from build123d import *

# Parameters (mm, degrees)
SKETCH1_R           = 2.39
SKETCH1_R_2         = 2.032
BOSS_EXTRUDE1_DEPTH = 3.175
FILLET1_R           = 9.525


with BuildPart() as part:
    # Sketch1 → Boss-Extrude1 (new body)
    with BuildSketch(Plane.XY):
        Polygon((-13.549562782, 51.201238591), (55.395997605, -32.358681046), (47.399630983, -77.865858829), (-38.635835903, 26.208991527), align=None)
        with Locations((-26.780789006, 24.707545021)):
            Circle(SKETCH1_R, mode=Mode.SUBTRACT)
        with Locations((24.186660888, -13.868436177)):
            Circle(SKETCH1_R_2, mode=Mode.SUBTRACT)
        with Locations((19.493324021, -31.017809025)):
            Circle(SKETCH1_R_2, mode=Mode.SUBTRACT)
        with Locations((39.76308397, -33.93171218)):
            Circle(SKETCH1_R_2, mode=Mode.SUBTRACT)
        with Locations((35.069747103, -51.081085027)):
            Circle(SKETCH1_R_2, mode=Mode.SUBTRACT)
    extrude(amount=BOSS_EXTRUDE1_DEPTH)

    # Fillet1
    fillet1_edges = [part.edges().sort_by_distance(p)[0] for p in [
        (-13.549562782, 51.201238591, 1.5875),
        (55.395997605, -32.358681046, 1.5875),
        (47.399630983, -77.865858829, 1.5875),
        (-38.635835903, 26.208991527, 1.5875),
    ]]
    fillet(fillet1_edges, radius=FILLET1_R)


solid = part.part
Verification items for the finished model (mm, model axes). Give positions to 0.01 mm unless a question says otherwise; leave off trailing zeros. Order: outer loops, then holes, each group sorted by start corner. A loop starts at its lowest first (then second) coordinate and runs counter-clockwise, first axis right, second up. Notation, with made-up numbers: M 74,32.25 L 79,32.25 A22 ccw 79,57.25 Z; hole C -1.75,-18 d1. An arc over 180 degrees is marked long. Answer as a JSON object with one key per item and string values. Group by question number.
1) Depth check by flat-ended pin: pin 1 Ø3.5 at (x, y) = (19.49, -31.02) entering from +Z; pin 2 Ø1.5 at (y, z) = (32, 2.5) entering from +X; pin 3 Ø1 at (x, z) = (7.5, 2.5) entering from +Y; pin 4 Ø6.5 at (x, y) = (39.76, -33.93) entering from +Z (3 decimals). Enter the tip coordinate at first touch or a pass-through.
2) Cross-section at B-B (y = -2). Enter the section's corners in (x, z) (3 decimals).
3) Cross-section at A-A (z = 2.4). Enter the section's corners in (x, y) (3 decimals), then the cut area to 3 significant figures.
4) Mould release check, pull along X, two halves, no side actions. Record for faces 1 (the face through (-13.664, 46.577, 1.61)), 2 (the face through (1.043, -21.79, 1.565)), 3 (the face through (20.43, -32.82, 1.57)): released by +X, released by -X, zero draft, split by the parting line, or undercut.
5) Scan lines: line 1 along X through (y, z) = (-13.5, 2.5); line 2 along X through (y, z) = (-14.5, 1.2); line 3 along X through (y, z) = (-24.5, 1.8). Record each from-to range of solid material in increasing order. Write a range as [from, to].
6) Cross-section at C-C (x = 14). Enter the section's corners in (y, z) (3 decimals).
Result sheet:
{
 "1": {"pin 1": "passes through", "pin 2": "stops at x = 2.91", "pin 3": "stops at y = 26.3", "pin 4": "stops at z = 3.175"},
 "2": {"outline": "M -15.316,0 L 30.347,0 L 30.347,3.175 L -15.316,3.175 Z"},
 "3": {"outline": "M -33.105,19.519 L 34.249,-61.958 A9.525 ccw 50.972,-57.538 L 54.636,-36.683 A9.525 ccw 52.602,-28.972 L -6.891,43.132 A9.525 ccw -20.961,43.818 L -32.486,32.335 A9.525 ccw Z; hole C -26.781,24.708 d4.78; hole C 19.493,-31.018 d4.064; hole C 24.187,-13.868 d4.064; hole C 35.07,-51.081 d4.064; hole C 39.763,-33.932 d4.064", "area": "4,080 mm2"},
 "4": {"face 1": "split by the parting line", "face 2": "released by -X", "face 3": "undercut"},
 "5": {"line 1": "x = [-5.81, 22.19], [26.18, 39.84]", "line 2": "x = [-4.98, 22.26], [26.12, 40.66]", "line 3": "x = [3.28, 48.91]"},
 "6": {"outline": "M -37.463,0 L 17.812,0 L 17.812,3.175 L -37.463,3.175 Z"}
}
